The listing builds one solid part. Answer for the finished solid, in the listing's coordinates (mm). Face numbers are marked on the shaded views. Coordinates: 2 decimals unless noted, no trailing zeros. Write each loop counter-clockwise with the first axis right and the second up, starting at its lowest first coordinate (ties: lowest second). Pieces come first, ordered by that corner, then holes.
```python
from build123d import *

# Parameters (mm, degrees)
SKETCH2_W                = 35
SKETCH2_H                = 35
BOSS_EXTRUDE1_DEPTH      = 10
SKETCH3_W                = 35
SKETCH3_H                = 35
SKETCH3_W_2              = 30
SKETCH3_H_2              = 30
BOSS_EXTRUDE2_DEPTH      = 15
SKETCH4_W                = 35
SKETCH4_H                = 35
BOSS_EXTRUDE3_DEPTH      = 15
CUT_EXTRUDE1_START       = -40
SKETCH5_R                = 3.05
CUT_EXTRUDE1_DEPTH       = 40
BOSS_EXTRUDE4_DEPTH      = 10
BOSS_EXTRUDE4_DEPTH_BACK = 45
SKETCH6_W                = 7.5
SKETCH6_H                = 1.017843133
SKETCH6_H_2              = 1.2761833
SKETCH7_R                = 2.76
CUT_EXTRUDE2_DEPTH       = 10


with BuildPart() as part:
    # Sketch2 → Boss-Extrude1 (new body)
    with BuildSketch(Plane(origin=(0, 0, 0), x_dir=(1, 0, 0), z_dir=(0, 1, 0))):
        Rectangle(SKETCH2_W, SKETCH2_H)
    extrude(amount=BOSS_EXTRUDE1_DEPTH)


with BuildPart() as body_2:
    # Sketch3 → Boss-Extrude2 (new body)
    with BuildSketch(Plane(origin=(0, 10, 0), x_dir=(1, 0, 0), z_dir=(0, 1, 0))):
        Rectangle(SKETCH3_W, SKETCH3_H)
        Rectangle(SKETCH3_W_2, SKETCH3_H_2, mode=Mode.SUBTRACT)
    extrude(amount=BOSS_EXTRUDE2_DEPTH)


with BuildPart() as body_3:
    # Sketch4 → Boss-Extrude3 (new body)
    with BuildSketch(Plane(origin=(0, 25, 0), x_dir=(1, 0, 0), z_dir=(0, 1, 0))):
        Rectangle(SKETCH4_W, SKETCH4_H)
    extrude(amount=BOSS_EXTRUDE3_DEPTH)


with BuildPart() as cut_extrude1_tool:
    # Sketch5 → Cut-Extrude1 (new body)
    with BuildSketch(Plane(origin=(0, 40, 0), x_dir=(1, 0, 0), z_dir=(0, 1, 0)).offset(CUT_EXTRUDE1_START)):
        with Locations(Location((0, 0, 0), (0, 0, 270))):
            Circle(SKETCH5_R)
    extrude(amount=CUT_EXTRUDE1_DEPTH)


with BuildPart() as part_1:
    add(part.part)

    # Cut-Extrude1: cut by cut_extrude1_tool
    add(cut_extrude1_tool.part, mode=Mode.SUBTRACT)


with BuildPart() as body_3_1:
    add(body_3.part)

    # Cut-Extrude1: cut by cut_extrude1_tool
    add(cut_extrude1_tool.part, mode=Mode.SUBTRACT)

    # Sketch6 → Boss-Extrude4 (add, two sides: drawn at the far end of the back side and taken through both)
    with BuildSketch(Plane(origin=(0, 0, -17.5), x_dir=(-1, 0, 0), z_dir=(0, 0, -1)).offset(-BOSS_EXTRUDE4_DEPTH_BACK)):
        with Locations((-13.75, 25.508921566)):
            Rectangle(SKETCH6_W, SKETCH6_H)
        with Locations((13.75, 25.63809165)):
            Rectangle(SKETCH6_W, SKETCH6_H_2)
    extrude(amount=BOSS_EXTRUDE4_DEPTH + BOSS_EXTRUDE4_DEPTH_BACK)

    # Sketch7 → Cut-Extrude2 (cut)
    with BuildSketch(Plane(origin=(0, 26.2761833, 0), x_dir=(1, 0, 0), z_dir=(0, 1, 0))):
        with Locations(Location((-13.75, 22.5, 0), (0, 0, 270))):
            Circle(SKETCH7_R)
        with Locations(Location((13.75, 22.5, 0), (0, 0, 270))):
            Circle(SKETCH7_R)
        with Locations(Location((13.75, -22, 0), (0, 0, 270))):
            Circle(SKETCH7_R)
        with Locations(Location((-13.75, -22, 0), (0, 0, 270))):
            Circle(SKETCH7_R)
    extrude(amount=-CUT_EXTRUDE2_DEPTH, mode=Mode.SUBTRACT)


solid = body_3_1.part
```
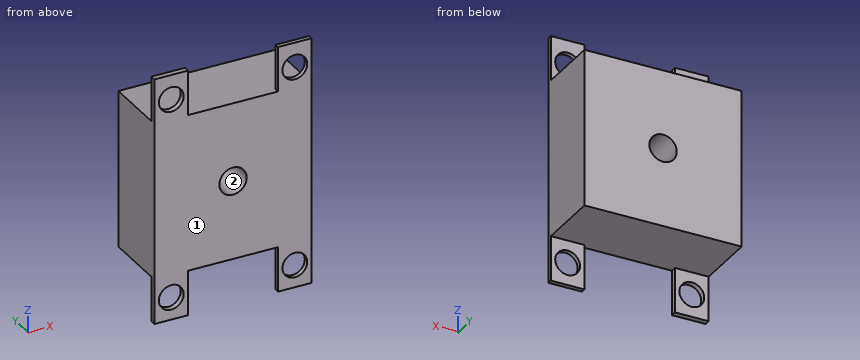
(1) Section A-A, the plane x = 13.75 is taken. Write down the section's boundary in (y, z), plus the area to 3 significant figures.
(2) Section C-C, the plane z = 0 is taken. Write down the section's boundary in (x, y).
(3) Find the intervals of material crossed by probe 1 along X at (y, z) = (25.45, -22.5); probe 2 along X at (y, z) = (36.5, 0), in increasing order.
(4) Section B-B, the plane x = 0 is taken. Write down the section's boundary in (y, z).
(5) Each of these flat-tipped pins is pushed along its axis until it touches: pin 1 (8 mm diameter, centred on x = 15.5, z = 21, fed in from +Y); pin 2 (7.5 mm diameter, centred on x = -7.5, y = 35, fed in from +Z); pin 3 (5 mm diameter, centred on x = 0, z = 0, fed in from +Y); pin 4 (4 mm diameter, centred on x = -14.5, z = -20.5, fed in from +Y). Where does it stop, or does it pass through?
(6) Section D-D, the plane y = 29.5 is taken. Write down the section's boundary in (x, z).
(7) For a pull along Z with two mould halves and no side action, classify the marked faces 1 and 2 as pulls with the +Z half, pulls with the -Z half, needs draft (parallel to the pull), parting line crosses it, or undercut.
Solution:
1. outline: (25, -27.5) - (26.02, -27.5) - (26.02, -25.26) - (25, -25.26) - close; (25, -19.74) - (26.02, -19.74) - (26.02, -17.5) - (40, -17.5) - (40, 17.5) - (26.02, 17.5) - (26.02, 19.24) - (25, 19.24) - close; (25, 24.76) - (26.02, 24.76) - (26.02, 27.5) - (25, 27.5) - close
1. area: 534 mm2
2. outline: (-17.5, 25) - (-3.05, 25) - (-3.05, 40) - (-17.5, 40) - close; (3.05, 25) - (17.5, 25) - (17.5, 40) - (3.05, 40) - close
3. probe 1: x = -17.5 to -16.51, -10.99 to -10, 10 to 10.99, 16.51 to 17.5
3. probe 2: x = -17.5 to -3.05, 3.05 to 17.5
4. outline: (25, -17.5) - (40, -17.5) - (40, -3.05) - (25, -3.05) - close; (25, 3.05) - (40, 3.05) - (40, 17.5) - (25, 17.5) - close
5. pin 1: stops at y = 40
5. pin 2: stops at z = 17.5
5. pin 3: passes through
5. pin 4: stops at y = 26.28
6. outline: (-17.5, -17.5) - (17.5, -17.5) - (17.5, 17.5) - (-17.5, 17.5) - close; hole circle Ø6.1 at (0, 0)
7. face 1: needs draft
7. face 2: undercut
